The listing builds one solid part. Answer for the finished solid, in the listing's coordinates (mm). Face numbers are marked on the shaded views. A direction names the side the tool comes from. Give positions to 0.01 mm unless a question says otherwise; leave off trailing zeros. Loops run counter-clockwise (first coordinate to the right, second up) from the corner with the lowest first, then second, coordinate; pieces in that order, holes last.
Item 1: Section D-D, the plane z = 11.25 is taken. Give the vertices of the cut face in (x, y) (3 decimals), and give its area (3 significant figures).
Item 2: Section A-A, the plane z = 0 is taken. Give the vertices of the cut face in (x, y) (3 decimals).
Item 3: A tool of negligible diameter and unlimited length cuts with its end or side. For the marked faces 1, 2 and 3, from which of +Z, -Z, +X, -X, +Y, -Y can it reach the whole face along a straight path? Write none if from no direction.
Item 4: Each of these flat-tipped pins is pushed along its axis until it touches: pin 1 Ø1.5 at (x, y) = (7.5, -25) entering from -Z; pin 2 Ø4 at (x, y) = (-1, -9) entering from -Z (3 decimals); pin 3 Ø4 at (x, y) = (-1, -38) entering from +Z. Where does it stop, or does it pass through?
Item 5: Section C-C, the plane y = -49 is taken. Give the vertices of the cut face in (x, z), and give its area (3 significant figures).
Item 6: Section B-B, the plane x = 0 is taken. Give the vertices of the cut face in (y, z) (3 decimals), and give its area (3 significant figures).
Item 7: Consider line 1 along Z through (x, y) = (0, -10.5) (3 decimals); line 2 along Z through (x, y) = (0, -28); line 3 along Y through (x, z) = (11, 4) (3 decimals). Determine where each line is inside the solid, lowest interval first.
Item 8: The mould has two halves that part along Z. Classify the marked faces 4, 5 and 6: pulls with the +Z half, pulls with the -Z half, needs draft (parallel to the pull), parting line crosses it, or undercut.
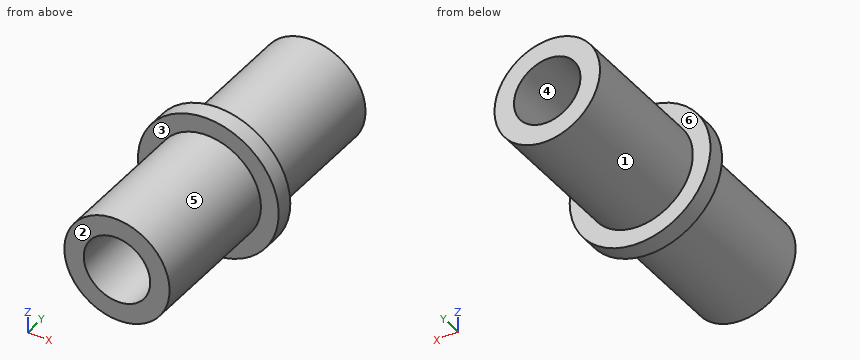
from build123d import *

# Parameters (mm, degrees)
F0_R     = 9.525
F0_R_2   = 6
F1_DEPTH = 25.4
F2_R     = 12.7
F2_R_2   = 9.525
F2_R_3   = 6
F3_DEPTH = 3.175
F4_R     = 9.5
F4_R_2   = 6
F5_DEPTH = 25


with BuildPart() as f1:
    # F0 (on Front) → F1 (new body)
    with BuildSketch(Plane.XZ):
        Circle(F0_R)
        Circle(F0_R_2, mode=Mode.SUBTRACT)
    extrude(amount=F1_DEPTH)

    # F2 (on face) → F3 (join)
    with BuildSketch(Plane.XZ.offset(25.4)):
        Circle(F2_R)
        Circle(F2_R_2, mode=Mode.SUBTRACT)
        Circle(F2_R_2)
        Circle(F2_R_3, mode=Mode.SUBTRACT)
    extrude(amount=F3_DEPTH)

    # F4 (on face) → F5 (join)
    with BuildSketch(Plane.XZ.offset(28.575)):
        Circle(F4_R)
        Circle(F4_R_2, mode=Mode.SUBTRACT)
    extrude(amount=F5_DEPTH)


solid = f1.part
Worked answers:
1. outline: (-5.893, -28.575) - (5.893, -28.575) - (5.893, -25.4) - (-5.893, -25.4) - close
1. area: 37.4 mm2
2. outline: (-12.7, -28.575) - (-9.5, -28.575) - (-9.5, -53.575) - (-6, -53.575) - (-6, 0) - (-9.525, 0) - (-9.525, -25.4) - (-12.7, -25.4) - close; (6, -53.575) - (9.5, -53.575) - (9.5, -28.575) - (12.7, -28.575) - (12.7, -25.4) - (9.525, -25.4) - (9.525, 0) - (6, 0) - close
3. face 1: +Y
3. face 2: +Z, -Z, +X, -X, -Y
3. face 3: -Y
4. pin 1: stops at z = -10.68
4. pin 2: stops at z = -9.525
4. pin 3: stops at z = 9.5
5. outline: circle Ø19 at (0, 0); hole circle Ø12 at (0, 0)
5. area: 170 mm2
6. outline: (-53.575, -9.5) - (-28.575, -9.5) - (-28.575, -12.7) - (-25.4, -12.7) - (-25.4, -9.525) - (0, -9.525) - (0, -6) - (-53.575, -6) - close; (-53.575, 6) - (0, 6) - (0, 9.525) - (-25.4, 9.525) - (-25.4, 12.7) - (-28.575, 12.7) - (-28.575, 9.5) - (-53.575, 9.5) - close
6. area: 397 mm2
7. line 1: z = -9.525 to -6, 6 to 9.525
7. line 2: z = -12.7 to -6, 6 to 12.7
7. line 3: y = -28.575 to -25.4
8. face 4: undercut
8. face 5: parting line crosses it
8. face 6: needs draft
